Design review of the part shown in the three views and the two pictorial views. Dimensions are in mm from the part's minimum x, y and z. A direction names the side the tool comes from. Round coordinates to 2 decimals unless told otherwise and drop trailing zeros. Order: outer loops, then holes, each group sorted by start corner. A loop starts at its lowest first (then second) coordinate and runs counter-clockwise, first axis right, second up.
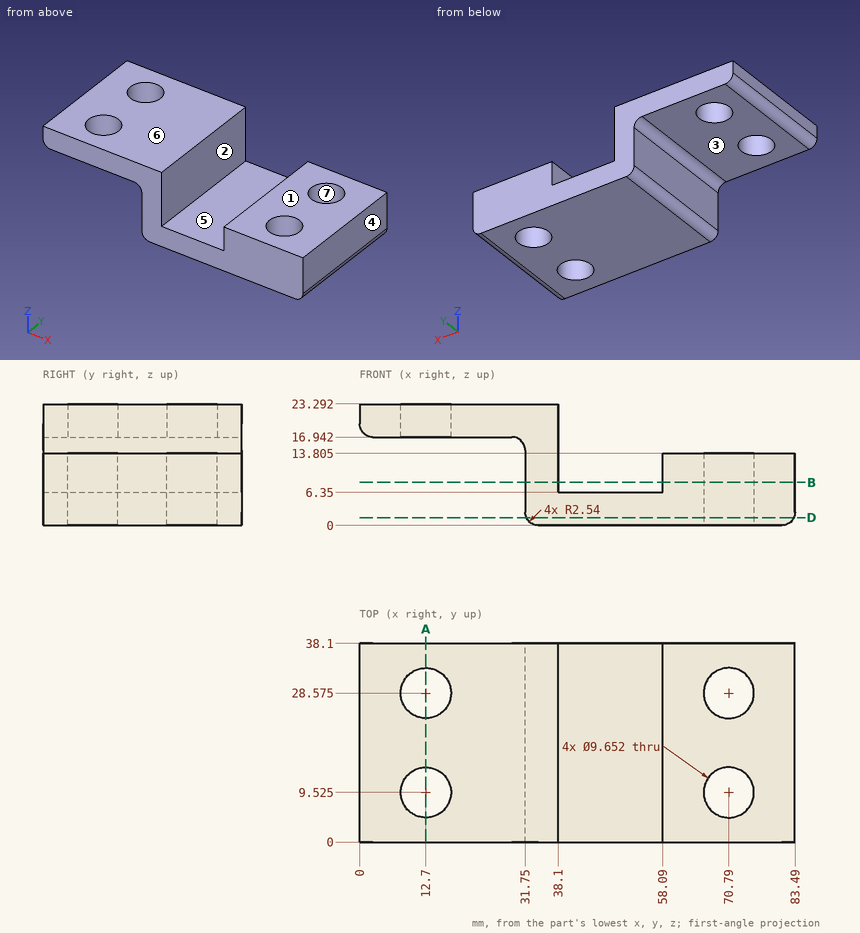
1) Take a section at A-A on x = 12.7. Give the boundary of the cut face in (y, z), plus the area to 3 significant figures.
Results:
outline: (0, 16.94) - (4.7, 16.94) - (4.7, 23.29) - (0, 23.29) - close; (14.35, 16.94) - (23.75, 16.94) - (23.75, 23.29) - (14.35, 23.29) - close; (33.4, 16.94) - (38.1, 16.94) - (38.1, 23.29) - (33.4, 23.29) - close
area: 119 mm2
2) Take a section at B-B on z = 8.25. State how many separate pieces and enclosed holes the cut face has, plus the area to 3 significant figures.
Results:
separate pieces: 2
enclosed holes: 2
area: 1,060 mm2
3) Take a section at D-D on z = 1.5. Give the boundary of the cut face in (x, y) (1 decimal), plus the area to 3 significant figures.
Results:
outline: (32, 0) - (83.3, 0) - (83.3, 38.1) - (32, 38.1) - close; hole circle Ø9.7 at (70.8, 9.5); hole circle Ø9.7 at (70.8, 28.6)
area: 1,810 mm2
4) To check wall thickness, follow line 1 along Y through (x, z) = (12.7, 21); line 2 along X through (y, z) = (26.5, 6.75); line 3 along X through (y, z) = (36.5, 8). State the ranges of each line that lie inside material, in increasing order.
Results:
line 1: y = 0 to 4.7, 14.35 to 23.75, 33.4 to 38.1
line 2: x = 31.75 to 38.1, 58.09 to 66.43, 75.15 to 83.49
line 3: x = 31.75 to 38.1, 58.09 to 83.49
5) The part is to be moulded in two halves that separate along X. For the marked faces 4, 5, 6 and 7, say which applies: released by +X, released by -X, zero draft, split by the parting line, or undercut.
Results:
face 4: released by +X
face 5: undercut
face 6: zero draft
face 7: undercut
6) For the marked faces 1, 2 and 3, list the 3-axis set-ups (+Z, -Z, +X, -X, +Y, -Y) from which the entire face can be reached by the end or side of a thin tool; tool diameter is ignored.
Results:
face 1: +Z, +X, +Y, -Y
face 2: +Z, +Y, -Y
face 3: -Z, -X, +Y, -Y
7) Clearance check with flat-ended pins moving along their axes: P1, Ø12.5, axis at x = 66.5, y = 16, coming from the +Z side (3 decimals); P2, Ø1, axis at x = 40, y = 20, coming from the +Z side; P3, Ø9.5, axis at y = 16.5, z = 9, coming from the -X side. State where each tip first meets the part, or that it passes through.
Results:
P1: stops at z = 13.805
P2: stops at z = 6.35
P3: stops at x = 31.75
